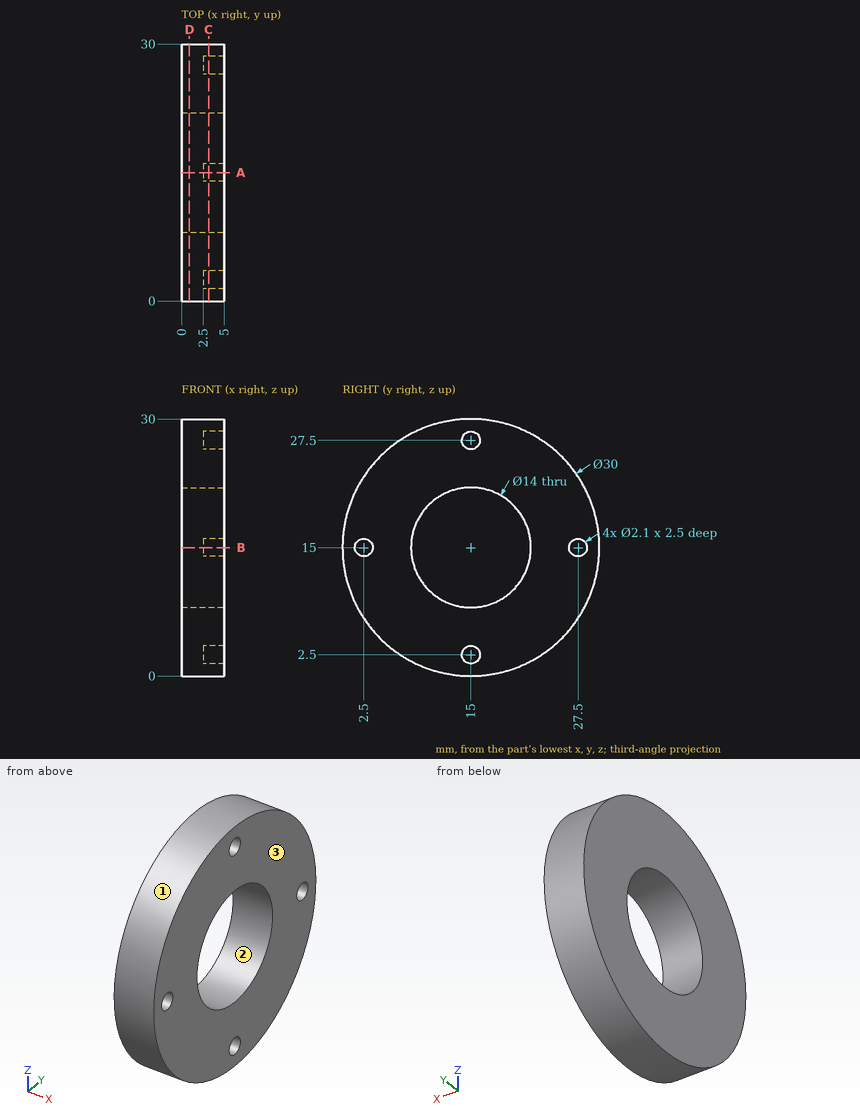
Could you check a few things on this drawing? It's one solid part, dimensions in mm from its lowest x, y, z. Coordinates: 2 decimals unless noted, no trailing zeros. Write each loop counter-clockwise with the first axis right and the second up, starting at its lowest first coordinate (ties: lowest second). Pieces come first, ordered by that corner, then holes.
1) If we section it at D-D (x = 0.9): List the corners of the cut face in (y, z) for me, plus the area to 3 significant figures.
Filled in:
outline: circle Ø30 at (15, 15); hole circle Ø14 at (15, 15)
area: 553 mm2
2) I'm going to push flat-ended pins straight in: pin 1 (3 mm diameter, centred on x = 2.5, y = 6.5, fed in from -Z); pin 2 (0.6 mm diameter, centred on y = 27, z = 15.5, fed in from +X); pin 3 (1.5 mm diameter, centred on x = 2, z = 17.5, fed in from -Y). Where does each tip first touch, or does it pass through?
Filled in:
pin 1: stops at z = 1.73
pin 2: stops at x = 2.5
pin 3: stops at y = 0.1
3) If we section it at A-A (y = 15): List the corners of the cut face in (x, z) for me, plus the area to 3 significant figures.
Filled in:
outline: (0, 0) - (5, 0) - (5, 1.45) - (2.5, 1.45) - (2.5, 3.55) - (5, 3.55) - (5, 8) - (0, 8) - close; (0, 22) - (5, 22) - (5, 26.45) - (2.5, 26.45) - (2.5, 28.55) - (5, 28.55) - (5, 30) - (0, 30) - close
area: 69.5 mm2
4) If I drill on line 1 (Y direction, x = 2.2, z = 15); line 2 (Y direction, x = 3.55, z = 3); line 3 (X direction, y = 27, z = 14.25), over which ranges is the centre line in solid material (lowest first)?
Filled in:
line 1: y = 0 to 8, 22 to 30
line 2: y = 6 to 14.08, 15.92 to 24
line 3: x = 0 to 2.5
5) If we section it at C-C (x = 3.15): List the corners of the cut face in (y, z) for me, plus the area to 3 significant figures.
Filled in:
outline: circle Ø30 at (15, 15); hole circle Ø2.1 at (2.5, 15); hole circle Ø14 at (15, 15); hole circle Ø2.1 at (15, 2.5); hole circle Ø2.1 at (15, 27.5); hole circle Ø2.1 at (27.5, 15)
area: 539 mm2
6) Thinking about a two-plate mould opening in Z: for the marked faces 1, 2 and 3, which applies, +Z half, -Z half, draft (parallel to the pull), parting line (faces both ways), or undercut?
Filled in:
face 1: parting line
face 2: undercut
face 3: draft
